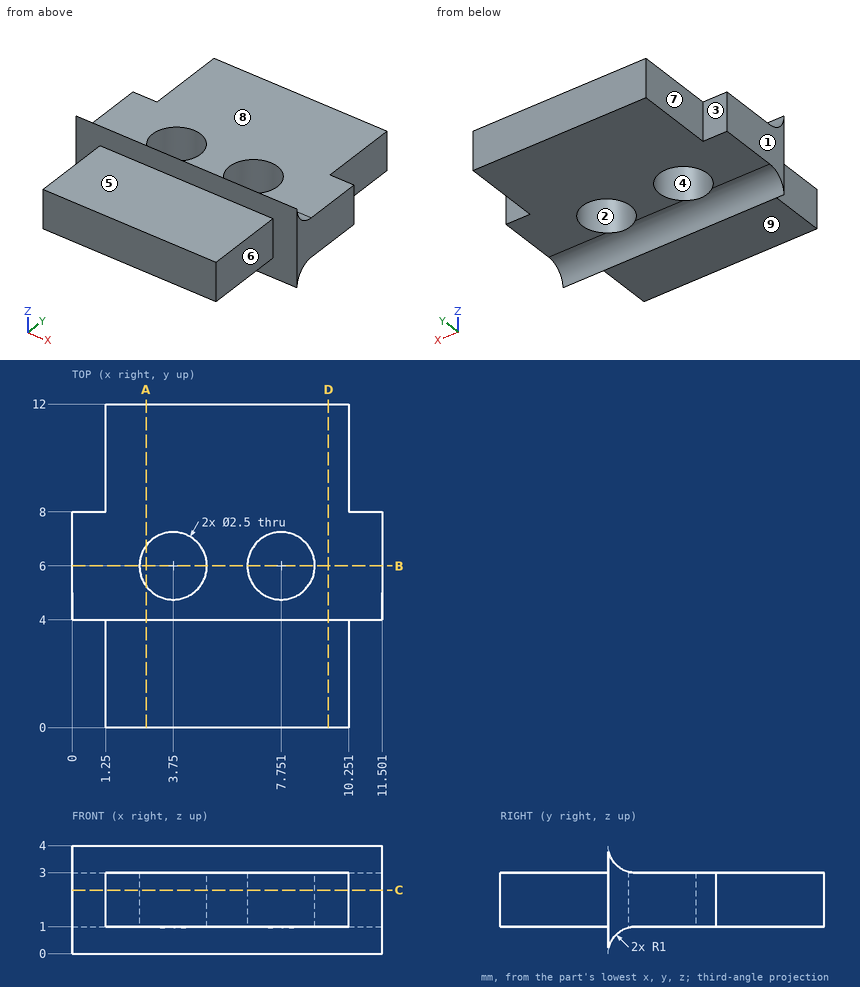
Geometry: see drawing. Coordinates: mm, zero at the bounding-box minimum. A direction names the side the tool comes from. Round coordinates to 2 decimals unless told otherwise and drop trailing zeros. Loops run counter-clockwise (first coordinate to the right, second up) from the corner with the lowest first, then second, coordinate; pieces in that order, holes last.
(1) Pull-direction query (Y, two-part tool) for the marked faces 1, 2, 3 and 4; classes: +Y half, -Y half, draft (parallel to the pull), parting line (faces both ways), or undercut.
From the geometry:
face 1: draft
face 2: undercut
face 3: +Y half
face 4: undercut
(2) Section query C-C (z = 2.35). Output: boundary loops of the cut face in (x, y).
From the geometry:
outline: (0, 4) - (1.25, 4) - (1.25, 0) - (10.25, 0) - (10.25, 4) - (11.5, 4) - (11.5, 8) - (10.25, 8) - (10.25, 12) - (1.25, 12) - (1.25, 8) - (0, 8) - close; hole circle Ø2.5 at (3.75, 6); hole circle Ø2.5 at (7.75, 6)
(3) Access query for the marked faces 5, 6, 7, 8 and 9. Directions: +Z, -Z, +X, -X, +Y, -Y. A direction counts if a zero-diameter tool reaches every point of the face in a straight line with its end or side. Return the directions, or none.
From the geometry:
face 5: +Z, +X, -X, -Y
face 6: +Z, -Z, +X, -Y
face 7: +Z, -Z, -X, +Y
face 8: +Z, +X, -X, +Y
face 9: -Z, +X, -X, -Y
(4) Section query B-B (y = 6). Output: boundary loops of the cut face in (x, z), and give its area (3 significant figures).
From the geometry:
outline: (0, 1) - (2.5, 1) - (2.5, 3) - (0, 3) - close; (5, 1) - (6.5, 1) - (6.5, 3) - (5, 3) - close; (9, 1) - (11.5, 1) - (11.5, 3) - (9, 3) - close
area: 13.0 mm2
(5) Section query A-A (x = 2.75). Output: boundary loops of the cut face in (y, z), and give its area (3 significant figures).
From the geometry:
outline: (0, 1) - (4, 1) - (4, 0) arc R1 cw to (5, 1) - (5.25, 1) - (5.25, 3) - (5, 3) arc R1 cw to (4, 4) - (4, 3) - (0, 3) - close; (6.75, 1) - (12, 1) - (12, 3) - (6.75, 3) - close
area: 21.4 mm2
(6) Contact query for flat-ended pins moving along their axis: pin 1 Ø5.5 at (x, y) = (6.5, 9) entering from +Z; pin 2 Ø1.6 at (y, z) = (9.5, 1.5) entering from -X; pin 3 Ø5.5 at (x, y) = (6, 7.5) entering from -Z. Output: stop coordinate, or through.
From the geometry:
pin 1: stops at z = 3
pin 2: stops at x = 1.25
pin 3: stops at z = 0.97
(7) Material intervals for probe 1 along X at (y, z) = (6, 1.85); probe 2 along Y at (x, z) = (3.75, 1.9); probe 3 along X at (y, z) = (5.25, 2.5), sorted ascending.
From the geometry:
probe 1: x = 0 to 2.5, 5 to 6.5, 9 to 11.5
probe 2: y = 0 to 4.75, 7.25 to 12
probe 3: x = 0 to 2.75, 4.75 to 6.75, 8.75 to 11.5
(8) Section query D-D (x = 9.5). Output: boundary loops of the cut face in (y, z), and give its area (3 significant figures).
From the geometry:
outline: (0, 1) - (4, 1) - (4, 0) arc R1 cw to (5, 1) - (12, 1) - (12, 3) - (5, 3) arc R1 cw to (4, 4) - (4, 3) - (0, 3) - close
area: 24.4 mm2
